Here's how the part is built. I have some questions about the finished solid (model axes, mm). Round coordinates to 2 decimals unless told otherwise and drop trailing zeros. Order: outer loops, then holes, each group sorted by start corner. A loop starts at its lowest first (then second) coordinate and runs counter-clockwise, first axis right, second up. Notation, with made-up numbers: M 65,84.25 L 90,84.25 A17 cw 90,98.25 Z; hole C -15,64.25 d2. An arc over 180 degrees is marked long. Write item = value, one per line. Start each with the question number.
Item 1: I'm going to push flat-ended pins straight in: P1, Ø2.5, axis at x = 1391.92, z = -136.92, coming from the +Y side; P2, Ø4, axis at y = -4.5, z = -101, coming from the -X side; P3, Ø6, axis at x = 649, y = -2.5, coming from the -Z side. Where does each tip first touch, or does it pass through?
Item 2: Please list where these lines run through material, in increasing order: L1, parallel to Z at x = 1099.82, y = -7.75 (3 decimals); L2, parallel to Z at x = 792.48, y = -8.75; L3, parallel to X at y = -3.25, z = 195.58 (3 decimals).
Item 3: I want a section at B-B, the plane y = -6.25. State how many separate pieces and enclosed holes the cut face has, plus the area to 3 significant figures.
Item 4: I want a section at A-A, the plane x = 203. List the corners of the cut face in (y, z) for me, plus the area to 3 significant figures.
```python
from build123d import *

# Parameters (mm, degrees)
F1_DEPTH = 12.7
F2_SIZE  = 25.4
F4_D     = 3.96875
F6_D     = 6.35
F8_D     = 4.826


with BuildPart() as f1:
    # F0 (on Front) → F1 (new body)
    with BuildSketch(Plane.XZ):
        with BuildLine():
            Line((0, 254), (0, 0))
            Line((0, 0), (635, 0))
            ThreePointArc((635, 0), (688.881537, -22.318463), (711.2, -76.2))
            Line((711.2, -76.2), (711.2, -154.3812))
            Line((711.2, -154.3812), (1473.2, -154.3812))
            Line((1473.2, -154.3812), (1473.2, 408.3812))
            Line((1473.2, 408.3812), (711.2, 408.3812))
            Line((711.2, 408.3812), (711.2, 330.2))
            ThreePointArc((711.2, 330.2), (688.881537, 276.318463), (635, 254))
            Line((635, 254), (0, 254))
        make_face()
    extrude(amount=F1_DEPTH)

    # F2
    f2_edges = [f1.edges().sort_by_distance(p)[0] for p in [
        (711.2, -6.35, 408.3812),
        (1473.2, -6.35, 408.3812),
        (1473.2, -6.35, -154.3812),
        (711.2, -6.35, -154.3812),
        (0, -6.35, 0),
        (0, -6.35, 254),
    ]]
    chamfer(f2_edges, length=F2_SIZE)

    # F4 (through all)
    with Locations(Plane.XZ.offset(12.7)):
        with Locations((767.08, 390.9314), (767.08, 348.0562), (792.48, 348.0562), (792.48, 390.9314), (767.08, -94.0562), (767.08, -136.9187), (792.48, -136.9187), (792.48, -94.0562), (1391.92, -94.0562), (1391.92, -136.9187), (1417.32, -136.9187), (1417.32, -94.0562), (1391.92, 348.0562), (1391.92, 390.9314), (1417.32, 390.9314), (1417.32, 348.0562)):
            Hole(F4_D / 2)

    # F6 (through all)
    with Locations(Plane.XZ.offset(12.7)):
        with Locations((1099.82, 195.58), (1099.82, 58.42), (1353.82, 58.42), (1353.82, 195.58)):
            Hole(F6_D / 2)

    # F8 (through all)
    with Locations(Plane.XZ.offset(12.7)):
        with Locations((10.16, 222.25), (27.94, 222.25), (10.16, 31.75), (27.94, 31.75), (734.06, 31.75), (751.84, 222.25), (734.06, 222.25), (751.84, 31.75)):
            Hole(F8_D / 2)


solid = f1.part
```
Filled in:
q1.P1 = through
q1.P2 = 711.2
q1.P3 = -1.92
q2.L1 = -154.381 to 55.245, 61.595 to 192.405, 198.755 to 408.381
q2.L2 = -154.38 to -138.9, -134.93 to -96.04, -92.07 to 346.07, 350.04 to 388.95, 392.92 to 408.38
q2.L3 = 0 to 1096.645, 1102.995 to 1350.645, 1356.995 to 1473.2
q3.separate_pieces = 1
q3.enclosed_holes = 28
q3.area = 610,000 mm^2
q4.outline = M -12.7,0 L 0,0 L 0,254 L -12.7,254 Z
q4.area = 3,230 mm^2
